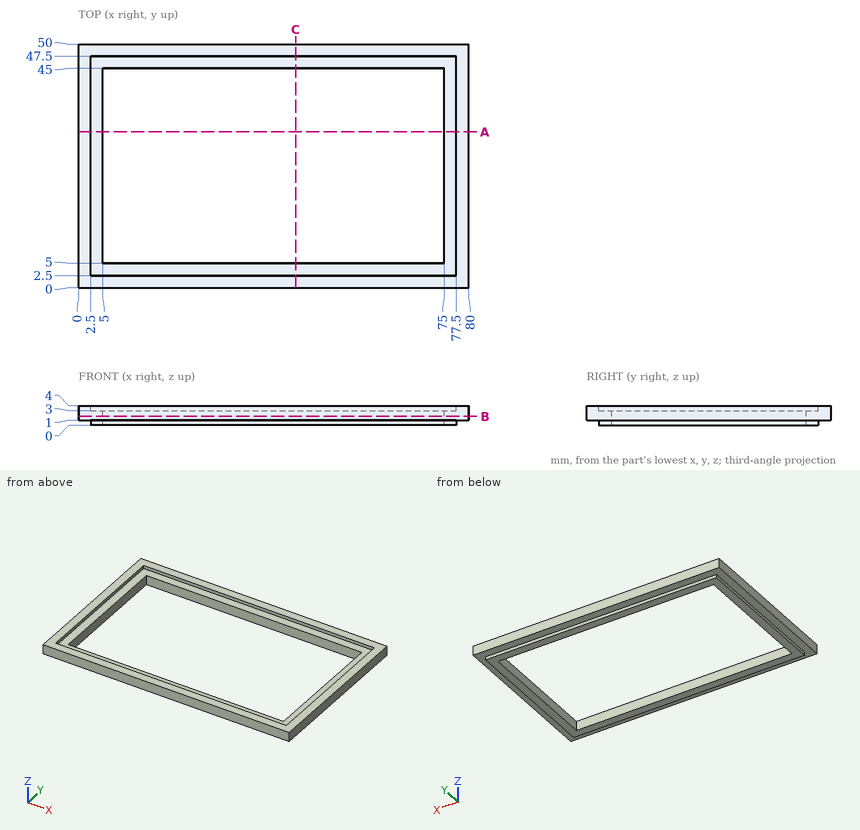
Geometry check sheet. Reference: drawing and pictorial views, mm from the part's lowest x, y, z. Round coordinates to 2 decimals unless told otherwise and drop trailing zeros. Loops run counter-clockwise (first coordinate to the right, second up) from the corner with the lowest first, then second, coordinate; pieces in that order, holes last.
1. Scan lines: probe 1 along X at (y, z) = (12, 2.35); probe 2 along Y at (x, z) = (34.5, 3.3); probe 3 along X at (y, z) = (45.5, 3.3). Record each from-to range of solid material in increasing order.
2. Sectioned sample at B-B on z = 1.85. Record the boundary of the cut face in (x, y).
3. Gauge pin test, flat ends, axial feed: pin 1 Ø2 at (x, y) = (24, 7) entering from +Z; pin 2 Ø0.8 at (y, z) = (24, 0.5) entering from -X; pin 3 Ø0.8 at (y, z) = (25, 0.5) entering from +X. Record the tip position at first contact, or that the pin passes through.
4. Sectioned sample at A-A on y = 32. Record the boundary of the cut face in (x, z), and give its area (3 significant figures).
5. Sectioned sample at C-C on x = 44.5. Record the boundary of the cut face in (y, z), and give its area (3 significant figures).
Recorded:
1. probe 1: x = 0 to 5, 75 to 80
1. probe 2: y = 0 to 2.5, 47.5 to 50
1. probe 3: x = 0 to 2.5, 77.5 to 80
2. outline: (0, 0) - (80, 0) - (80, 50) - (0, 50) - close; hole (5, 5) - (75, 5) - (75, 45) - (5, 45) - close
3. pin 1: passes through
3. pin 2: stops at x = 2.5
3. pin 3: stops at x = 77.5
4. outline: (0, 1) - (2.5, 1) - (2.5, 0) - (5, 0) - (5, 3) - (2.5, 3) - (2.5, 4) - (0, 4) - close; (75, 0) - (77.5, 0) - (77.5, 1) - (80, 1) - (80, 4) - (77.5, 4) - (77.5, 3) - (75, 3) - close
4. area: 30.0 mm2
5. outline: (0, 1) - (2.5, 1) - (2.5, 0) - (5, 0) - (5, 3) - (2.5, 3) - (2.5, 4) - (0, 4) - close; (45, 0) - (47.5, 0) - (47.5, 1) - (50, 1) - (50, 4) - (47.5, 4) - (47.5, 3) - (45, 3) - close
5. area: 30.0 mm2
